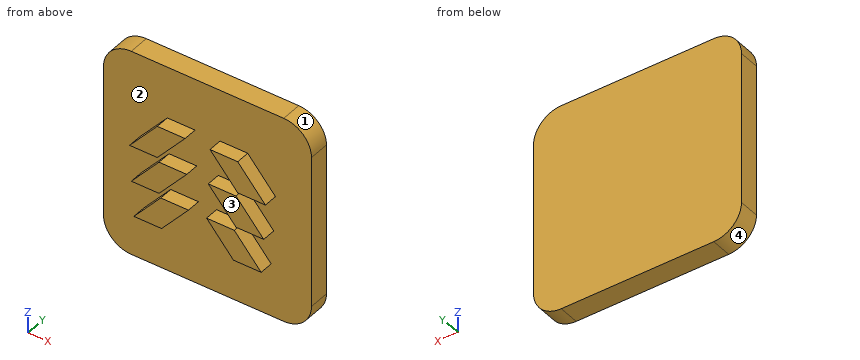
from build123d import *

# Parameters (mm, degrees)
F0_W     = 38.1
F0_H     = 38.1
F1_DEPTH = 3.81
F2_R     = 5.08
F4_DEPTH = 2.54


with BuildPart() as f1:
    # F0 (on Front) → F1 (new body)
    with BuildSketch(Plane.XZ):
        Rectangle(F0_W, F0_H)
    extrude(amount=F1_DEPTH)

    # F2
    f2_edges = [f1.edges().sort_by_distance(p)[0] for p in [
        (19.05, -1.905, 19.05),
        (-19.05, -1.905, 19.05),
        (-19.05, -1.905, -19.05),
        (19.05, -1.905, -19.05),
    ]]
    fillet(f2_edges, radius=F2_R)

    # F3 (on face) → F4 (join)
    with BuildSketch(Plane.XZ.offset(3.81)):
        Polygon((-7.366, 3.678485), (-2.286, 9.525), (-7.366, 9.525), (-12.446, 3.678485), align=None)
        Polygon((-1.973369, 2.942095), (-7.052271, 2.942095), (-12.133434, -2.905793), (-7.053434, -2.905793), align=None)
        Polygon((-1.659051, -3.629045), (-6.739051, -3.629045), (-11.663045, -9.296048), (-6.583045, -9.296048), align=None)
        Polygon((11.663045, -9.296048), (6.739051, -3.629045), (1.659051, -3.629045), (6.583045, -9.296048), align=None)
        Polygon((12.133434, -2.905793), (7.052271, 2.942095), (1.973369, 2.942095), (7.053434, -2.905793), align=None)
        Polygon((2.286, 9.525), (7.366, 3.678485), (12.446, 3.678485), (7.366, 9.525), align=None)
    extrude(amount=F4_DEPTH)


solid = f1.part
Input: part model. Units: mm. Frame: model coordinates. Face numbers are marked on the shaded views. Coordinates: 2 decimals unless noted, no trailing zeros. Loops run counter-clockwise (first coordinate to the right, second up) from the corner with the lowest first, then second, coordinate; pieces in that order, holes last. Notation, with made-up numbers: (15, 82) -> (33, 82) arc R23 cw to (33, 110) -> close; hole circle Ø7 at (4.5, 3.5). An arc over 180 degrees is marked (long way). One line per item, written item: value.
(1) Ray query, line 1 along Y through (x, z) = (-8, -17); line 2 along X through (y, z) = (-5, 2.5); line 3 along X through (y, z) = (-4, 1.5). Return the intervals inside material, ascending.
Answer below:
line 1: y = -3.81 to 0
line 2: x = -7.44 to -2.36, 2.36 to 7.44
line 3: x = -8.31 to -3.23, 3.23 to 8.31
(2) Pin query (flat end, axial travel): pin 1 Ø1.5 at (x, y) = (4, -4) entering from +Z; pin 2 Ø3 at (x, y) = (-8.5, -5.5) entering from -Z; pin 3 Ø1.3 at (x, y) = (3.5, -5) entering from +Z (3 decimals). Return the tip coordinate at first contact, or that it passes through.
Answer below:
pin 1: stops at z = 19.05
pin 2: stops at z = -9.3
pin 3: stops at z = 9.525
(3) Cut plane D-D (x = -3). Output: boundary loops of the cut face in (y, z) (3 decimals), then the cut area to 3 significant figures.
Answer below:
outline: (-6.35, -5.172) -> (-3.81, -5.172) -> (-3.81, -19.05) -> (0, -19.05) -> (0, 19.05) -> (-3.81, 19.05) -> (-3.81, 9.525) -> (-6.35, 9.525) -> (-6.35, 8.703) -> (-3.81, 8.703) -> (-3.81, 2.942) -> (-6.35, 2.942) -> (-6.35, 1.76) -> (-3.81, 1.76) -> (-3.81, -3.629) -> (-6.35, -3.629) -> close
area: 154 mm2
(4) Draft query along X for the marked faces 1, 2, 3 and 4. Return one class per face: pulls with the +X half, pulls with the -X half, needs draft (parallel to the pull), parting line crosses it, or undercut.
Answer below:
face 1: pulls with the +X half
face 2: undercut
face 3: needs draft
face 4: pulls with the -X half
(5) Cut plane C-C (z = 1). Output: boundary loops of the cut face in (x, y).
Answer below:
outline: (-19.05, -3.81) -> (-8.74, -3.81) -> (-8.74, -6.35) -> (-3.66, -6.35) -> (-3.66, -3.81) -> (3.66, -3.81) -> (3.66, -6.35) -> (8.74, -6.35) -> (8.74, -3.81) -> (19.05, -3.81) -> (19.05, 0) -> (-19.05, 0) -> close
(6) Cut plane B-B (y = -2.25). Output: boundary loops of the cut face in (x, z), then the cut area to 3 significant figures.
Answer below:
outline: (-19.05, -13.97) arc R5.08 ccw to (-13.97, -19.05) -> (13.97, -19.05) arc R5.08 ccw to (19.05, -13.97) -> (19.05, 13.97) arc R5.08 ccw to (13.97, 19.05) -> (-13.97, 19.05) arc R5.08 ccw to (-19.05, 13.97) -> close
area: 1,430 mm2
(7) Cut plane A-A (y = -5.5). Output: boundary loops of the cut face in (x, z) (3 decimals).
Answer below:
outline: (-12.446, 3.678) -> (-7.366, 3.678) -> (-2.286, 9.525) -> (-7.366, 9.525) -> close; (-12.133, -2.906) -> (-7.053, -2.906) -> (-1.973, 2.942) -> (-7.052, 2.942) -> close; (-11.663, -9.296) -> (-6.583, -9.296) -> (-1.659, -3.629) -> (-6.739, -3.629) -> close; (1.659, -3.629) -> (6.583, -9.296) -> (11.663, -9.296) -> (6.739, -3.629) -> close; (1.973, 2.942) -> (7.053, -2.906) -> (12.133, -2.906) -> (7.052, 2.942) -> close; (2.286, 9.525) -> (7.366, 3.678) -> (12.446, 3.678) -> (7.366, 9.525) -> close
